from build123d import *

# Parameters (mm, degrees)
SKETCH021_R             = 38.773757
PAD011_DEPTH            = 10
SKETCH024_R             = 17
PAD012_DEPTH            = 15
SKETCH023_R             = 7
HOLE007_DEPTH           = 33
SKETCH022_R             = 2.75
HOLE008_DEPTH           = 41.347633
HOLE008_TIPS_R          = 2.75
BODY010_PLACEMENT_ANGLE = 90


with BuildPart() as part:
    # Sketch021 → Pad011 (new body)
    with BuildSketch(Plane.XY):
        with Locations((-46.112587, 35.075455)):
            Circle(SKETCH021_R)
    extrude(amount=PAD011_DEPTH)

    # Sketch024 (on Face2 of Pad011) → Pad012 (join)
    with BuildSketch(Plane(origin=(0, 0, 0), x_dir=(1, 0, 0), z_dir=(0, 0, -1))):
        with Locations((-47, -36)):
            Circle(SKETCH024_R)
    extrude(amount=PAD012_DEPTH)

    # Sketch023 (on Face5 of Pad012) → Hole007 (cut)
    with BuildSketch(Plane(origin=(0, 0, -15), x_dir=(1, 0, 0), z_dir=(0, 0, -1))):
        with Locations((-47.024734, -35.997555)):
            Circle(SKETCH023_R)
    extrude(amount=-HOLE007_DEPTH, mode=Mode.SUBTRACT)

    # Sketch022 → Hole008 (cut)
    with BuildSketch(Plane.YZ):
        with Locations((35.974483, -6.968689)):
            Circle(SKETCH022_R)
    extrude(amount=-HOLE008_DEPTH, mode=Mode.SUBTRACT)

    # Hole008 tips → Hole008 tip 1 section 0
    with BuildSketch(Plane.YZ.offset(-41.347633), mode=Mode.PRIVATE) as hole008_tip_1_s0:
        with Locations((35.974483, -6.968689)):
            Circle(HOLE008_TIPS_R)
    loft([hole008_tip_1_s0.sketch, Vertex(-43, 35.974483, -6.968689)], mode=Mode.SUBTRACT)


with BuildPart() as part_1:
    # Body010 placement: moved
    add(part.part.moved(Location((1, -55, -178))).rotate(Axis((1, -55, -178), (1, 0, 0)), BODY010_PLACEMENT_ANGLE))


solid = part_1.part
Design review of the part built by this model. Coordinates are the model's own, in mm. A direction names the side the tool comes from. Coordinates: 2 decimals unless noted, no trailing zeros. Order: outer loops, then holes, each group sorted by start corner. A loop starts at its lowest first (then second) coordinate and runs counter-clockwise, first axis right, second up.
Item 1: For line 1 (Y direction, x = -60, z = -157); line 2 (X direction, y = -61, z = -158); line 3 (X direction, y = -57, z = -137.5), list the stretches that pass through material, from the lowest coordinate up.
Item 2: Take a section at A-A, the plane x = -46. Write out the cut boundary in (y, z).
Item 3: The part is to be moulded in two halves that separate along Z. For faces 1 (the cylindrical face through (-53.518, -59.93, -180.776)), 2 (the flat face through (-46.2, -40, -134.7)), 3 (the cylindrical face through (-34.225, -46.978, -139.485)), say which applies: pulls with the +Z half, pulls with the -Z half, needs draft (parallel to the pull), parting line crosses it, or undercut.
Item 4: For faces 4 (the cylindrical face through (-48.213, -47.605, -158.855)), 5 (the flat face through (-46, -65, -151)), list the 3-axis set-ups (+Z, -Z, +X, -X, +Y, -Y) from which the entire face can be reached by the end or side of a thin tool; tool diameter is ignored.
Item 5: For pin 1 Ø5 at (y, z) = (-48.03, -142.03) entering from +X; pin 2 Ø1 at (x, y) = (-64, -55) entering from +Z; pin 3 Ø3 at (x, y) = (-40.5, -42.5) entering from -Z; pin 4 Ø2 at (x, z) = (-41.5, -139) entering from -Y, all flat-tipped, find the tip position at first contact; note any pin that passes through.
Item 6: Take a section at B-B, the plane y = -52. Write out the cut boundary in (x, z).
Item 7: Take a section at D-D, the plane y = -46.25. Write out the cut boundary in (x, z).
Item 8: Take a section at C-C, the plane z = -124. Write out the cut boundary in (x, y), then the cut area to 3 significant figures.
The answers:
1. line 1: y = -65 to -55
1. line 2: x = -80.84 to -9.39
1. line 3: x = -83.51 to -51.38, -40.66 to -6.72
2. outline: (-65, -181.69) - (-55, -181.69) - (-55, -159) - (-40, -159) - (-40, -149) - (-65, -149) - close; (-65, -135) - (-40, -135) - (-40, -125) - (-55, -125) - (-55, -104.16) - (-65, -104.16) - close
3. face 1: parting line crosses it
3. face 2: needs draft
3. face 3: undercut
4. face 4: +Y
4. face 5: +Z, -Z, +X, -X, -Y
5. pin 1: stops at x = -52.55
5. pin 2: stops at z = -108.79
5. pin 3: stops at z = -158.52
5. pin 4: passes through
6. outline: circle Ø34 at (-46, -142); hole circle Ø14 at (-46.02, -142)
7. outline: (-39.35, -144.12) arc R7 cw (long way) to (-39.34, -139.93) - (-29.13, -139.93) arc R17 ccw (long way) to (-29.13, -144.12) - close
8. outline: (-78.95, -65) - (-11.27, -65) - (-11.27, -55) - (-78.95, -55) - close
8. area: 677 mm2
